Model file for the job. Use its own axes, mm. A direction names the side the tool comes from. Give positions to 0.01 mm unless a question says otherwise; leave off trailing zeros. Loops run counter-clockwise (first coordinate to the right, second up) from the corner with the lowest first, then second, coordinate; pieces in that order, holes last. Notation, with made-up numbers: M -17,35 L -8,35 A33 cw -8,66 Z; hole C 25.25,27.5 d5. An arc over 180 degrees is marked long. Answer in a Markdown table with one row per item.
```python
from build123d import *

# Parameters (mm, degrees)
SKETCH_2_W          = 57
SKETCH_2_H          = 40.4
EXTRUDE_1_DEPTH     = 1.5
SKETCH_4_R          = 3
SKETCH_4_R_2        = 1.5
EXTRUDE_3_DEPTH     = 4
SKETCH_5_W          = 57
SKETCH_5_H          = 4.2
CUT_EXTRUDE_1_DEPTH = 2.5
SKETCH_6_W          = 1
SKETCH_6_H          = 32
EXTRUDE_4_DEPTH     = 1.5


with BuildPart() as part:
    # 草图2 → 凸台-拉伸1 (new body)
    with BuildSketch(Plane(origin=(0, 0, 0), x_dir=(1, 0, 0), z_dir=(0, 1, 0))):
        with Locations((3.861898857, -4.534326193)):
            Rectangle(SKETCH_2_W, SKETCH_2_H)
    extrude(amount=EXTRUDE_1_DEPTH)

    # 草图4 → 凸台-拉伸3 (add)
    with BuildSketch(Plane(origin=(0, 1.5, 0), x_dir=(1, 0, 0), z_dir=(0, 1, 0))):
        with Locations((-22.099370277, 7.765673807)):
            Circle(SKETCH_4_R)
        with Locations((-22.099370277, 7.765673807)):
            Circle(SKETCH_4_R_2, mode=Mode.SUBTRACT)
        with Locations((-22.138101143, -16.834326193)):
            Circle(SKETCH_4_R)
        with Locations((-22.138101143, -16.834326193)):
            Circle(SKETCH_4_R_2, mode=Mode.SUBTRACT)
        with Locations((29.861898857, -16.834326193)):
            Circle(SKETCH_4_R)
        with Locations((29.861898857, -16.834326193)):
            Circle(SKETCH_4_R_2, mode=Mode.SUBTRACT)
        with Locations((29.861898857, 7.765673807)):
            Circle(SKETCH_4_R)
        with Locations((29.861898857, 7.765673807)):
            Circle(SKETCH_4_R_2, mode=Mode.SUBTRACT)
    extrude(amount=EXTRUDE_3_DEPTH)

    # 草图5 → 切除-拉伸1 (cut, through all)
    with BuildSketch(Plane(origin=(0, 1.5, 0), x_dir=(1, 0, 0), z_dir=(0, 1, 0))):
        with Locations((3.861898857, 13.565673807)):
            Rectangle(SKETCH_5_W, SKETCH_5_H)
        with Locations((3.861898857, -22.634326193)):
            Rectangle(SKETCH_5_W, SKETCH_5_H)
    extrude(amount=-CUT_EXTRUDE_1_DEPTH, mode=Mode.SUBTRACT)

    # 草图6 → 凸台-拉伸4 (add)
    with BuildSketch(Plane(origin=(0, 1.5, 0), x_dir=(1, 0, 0), z_dir=(0, 1, 0))):
        with Locations((-25.138101143, -4.534326193)):
            Rectangle(SKETCH_6_W, SKETCH_6_H)
        with Locations((32.861898857, -4.534326193)):
            Rectangle(SKETCH_6_W, SKETCH_6_H)
    extrude(amount=-EXTRUDE_4_DEPTH)


solid = part.part
```
Q1. Saw through at C-C (z = -3.5). Give the cut face in (x, y).
Reported:
| item | result |
|---|---|
| outline | M -25.64,0 L 33.36,0 L 33.36,1.5 L -25.64,1.5 Z |
Q2. Drop a flat-ended pin along its axis: pin 1 (1 mm diameter, centred on x = -9, z = 11, fed in from +Y). Give the stop position or say it passes through.
Reported:
| item | result |
|---|---|
| pin 1 | y = 1.5 |
Q3. Probe probe 1 along X at (y, z) = (5.1, -6.5); probe 2 along X at (y, z) = (5.05, 15.5); probe 3 along Y at (x, z) = (13.5, 4). List the from-to ranges inside material, lowest first.
Reported:
| item | result |
|---|---|
| probe 1 | -24.82 to -22.9, -21.29 to -19.38, 27.14 to 29.06, 30.67 to 32.58 |
| probe 2 | -24.83 to -22.82, -21.45 to -19.45, 27.17 to 29.18, 30.55 to 32.55 |
| probe 3 | 0 to 1.5 |
Q4. 3-axis set-ups, long thin cutter, end or side, ignore diameter. For faces 1 (the face through (32.723, 3.472, 15.933)), 2 (the face through (-24, 5.5, 17)): which of +Z, -Z, +X, -X, +Y, -Y reach the whole face in a straight line?
Reported:
| item | result |
|---|---|
| face 1 | +Y |
| face 2 | +Z, -Z, +X, -X, +Y |
Q5. Saw through at D-D (z = 16). Give the cut face in (x, y).
Reported:
| item | result |
|---|---|
| outline | M -25.64,0 L 33.36,0 L 33.36,1.5 L 32.74,1.5 L 32.74,5.5 L 31.11,5.5 L 31.11,1.5 L 28.62,1.5 L 28.62,5.5 L 26.98,5.5 L 26.98,1.5 L -19.26,1.5 L -19.26,5.5 L -20.89,5.5 L -20.89,1.5 L -23.38,1.5 L -23.38,5.5 L -25.02,5.5 L -25.02,1.5 L -25.64,1.5 Z |
Q6. Saw through at B-B (x = -20). Give the cut face in (y, z), and give its area (3 significant figures).
Reported:
| item | result |
|---|---|
| outline | M 0,-11.47 L 1.5,-11.47 L 1.5,-9.91 L 5.5,-9.91 L 5.5,-5.62 L 1.5,-5.62 L 1.5,14.73 L 5.5,14.73 L 5.5,18.94 L 1.5,18.94 L 1.5,20.53 L 0,20.53 Z |
| area | 82.0 mm² |
Q7. Saw through at A-A (y = 4). Give the cut face in (x, z), and give its area (3 significant figures).
Reported:
| item | result |
|---|---|
| outline | C -22.14,16.83 d6; C -22.1,-7.77 d6; C 29.86,-7.77 d6; C 29.86,16.83 d6; hole C -22.14,16.83 d3; hole C -22.1,-7.77 d3; hole C 29.86,-7.77 d3; hole C 29.86,16.83 d3 |
| area | 84.8 mm² |
Q8. Mould opens along X. For faces 3 (the face through (30, 5.5, 15)), 4 (the face through (-19.277, 3.472, 15.933)), 5 (the face through (-23.637, 3.472, 16.768)), 6 (the face through (-25.638, 1, 5)) say: released by +X, released by -X, zero draft, split by the parting line, or undercut.
Reported:
| item | result |
|---|---|
| face 3 | zero draft |
| face 4 | undercut |
| face 5 | undercut |
| face 6 | released by -X |
